Source: three-view drawing plus pictorial views. Frame: mm from the lowest corner of the part. A direction names the side the tool comes from. Give positions to 0.01 mm unless a question says otherwise; leave off trailing zeros. Order: outer loops, then holes, each group sorted by start corner. A loop starts at its lowest first (then second) coordinate and runs counter-clockwise, first axis right, second up. Notation, with made-up numbers: (5.25, -3) -> (40.25, -3) arc R21 cw to (40.25, 20) -> close; hole circle Ø11 at (-16.5, 53.5). An arc over 180 degrees is marked (long way). Answer in a Markdown table with one row per item. Add a question column.
Q1. Set-up query: the marked faces 5 and 6. Return all of +Z, -Z, +X, -X, +Y, -Y with unobstructed straight access to the full face (end or side cutting, diameter ignored); none if empty.
Q2. Cut plane B-B on y = 11. Return the cut outline in (x, z).
Q3. Line query: line 1 along Y through (x, z) = (5.7, 3.1); line 2 along Y through (x, z) = (36, 3.65); line 3 along X through (y, z) = (25.5, 2.95). Output: solid intervals per line, ascending. Write a range as from..to.
Q4. Cut plane C-C on y = 24. Return the cut outline in (x, z).
Q5. Pull-direction query (X, two-part tool) for the marked faces 1, 2, 3 and 4; classes: +X half, -X half, draft (parallel to the pull), parting line (faces both ways), or undercut.
Q6. Contact query for a flat-ended pin moving along its axis: P1, Ø3, axis at x = 54.3, y = 11, coming from the +Z side. Output: stop coordinate, or through.
Q7. Cut plane A-A on x = 54.3. Return the cut outline in (y, z).
Q8. Cut plane D-D on x = 33. Return the cut outline in (y, z), and give its area (3 significant figures).
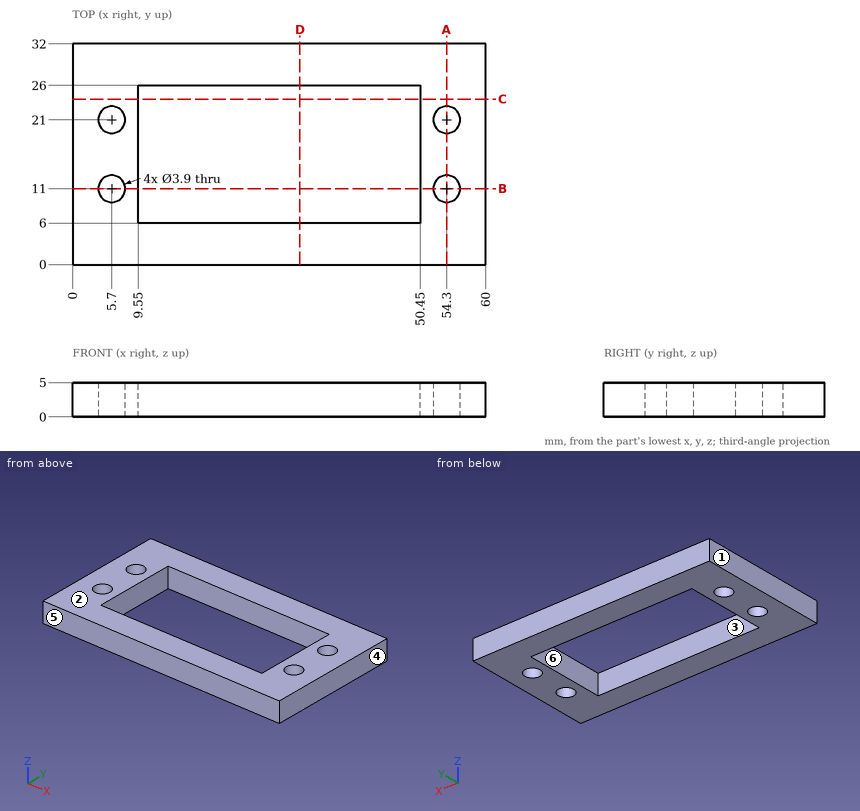
Completed:
| question | item | result |
|---|---|---|
| 1 | face 5 | +Z, -Z, +X, -X, -Y |
| 1 | face 6 | +Z, -Z |
| 2 | outline | (0, 0) -> (3.75, 0) -> (3.75, 5) -> (0, 5) -> close; (7.65, 0) -> (9.55, 0) -> (9.55, 5) -> (7.65, 5) -> close; (50.45, 0) -> (52.35, 0) -> (52.35, 5) -> (50.45, 5) -> close; (56.25, 0) -> (60, 0) -> (60, 5) -> (56.25, 5) -> close |
| 3 | line 1 | y = 0..9.05, 12.95..19.05, 22.95..32 |
| 3 | line 2 | y = 0..6, 26..32 |
| 3 | line 3 | x = 0..9.55, 50.45..60 |
| 4 | outline | (0, 0) -> (9.55, 0) -> (9.55, 5) -> (0, 5) -> close; (50.45, 0) -> (60, 0) -> (60, 5) -> (50.45, 5) -> close |
| 5 | face 1 | -X half |
| 5 | face 2 | draft |
| 5 | face 3 | undercut |
| 5 | face 4 | +X half |
| 6 | P1 | passes through |
| 7 | outline | (0, 0) -> (9.05, 0) -> (9.05, 5) -> (0, 5) -> close; (12.95, 0) -> (19.05, 0) -> (19.05, 5) -> (12.95, 5) -> close; (22.95, 0) -> (32, 0) -> (32, 5) -> (22.95, 5) -> close |
| 8 | outline | (0, 0) -> (6, 0) -> (6, 5) -> (0, 5) -> close; (26, 0) -> (32, 0) -> (32, 5) -> (26, 5) -> close |
| 8 | area | 60.0 mm² |
